Could you check a few things on this model? Use its own coordinates, in mm. Face numbers are marked on the shaded views. A direction names the side the tool comes from. Give positions to 0.01 mm unless a question says otherwise; leave off trailing zeros. Order: outer loops, then holes, each group sorted by start corner. A loop starts at its lowest first (then second) coordinate and runs counter-clockwise, first axis right, second up. Notation, with made-up numbers: (86, -8) -> (95, -8) arc R17 cw to (95, 13) -> close; hole circle Ø10 at (-38, 74.25). An arc over 180 degrees is marked (long way). Answer as CSV lines item,"result". Start each with the question number.
(1) I want a section at C-C (z = 21). Please give me the cut outline in (x, y), plus the area to 3 significant figures.
(2) We'd pull the mould along Z, two halves only. Please class the marked faces 3, 4, 5 and 6: released by +Z, released by -Z, zero draft, split by the parting line, or undercut.
(3) I want a section at A-A (y = 0). Please give me the cut outline in (x, z), plus the area to 3 significant figures.
(4) I need wall thicknesses on L1, parallel to Y at x = 0, z = 30.5; L2, parallel to Y at x = 0, z = 16; L3, parallel to Z at x = 14.5, y = -2.5. Which ranges of each line are inside material? Lowest first, please.
(5) I want a section at D-D (y = -11). Please give me the cut outline in (x, z), plus the area to 3 significant figures.
(6) Will these pins go through, and if not, where does the flat tip stop? pin 1 Ø5 at (y, z) = (8.5, 18.5) entering from +X; pin 2 Ø1.5 at (x, z) = (-8.5, 9.5) entering from +Y; pin 3 Ø1.5 at (x, z) = (6.5, 12.5) entering from +Y.
(7) On a 3-axis mill with a long thin cutter (end or side, diameter ignored), from which of +Z, -Z, +X, -X, +Y, -Y can I reach the whole of each face in a straight line? I mean the marked faces 1 and 2. Say none if no direction works.
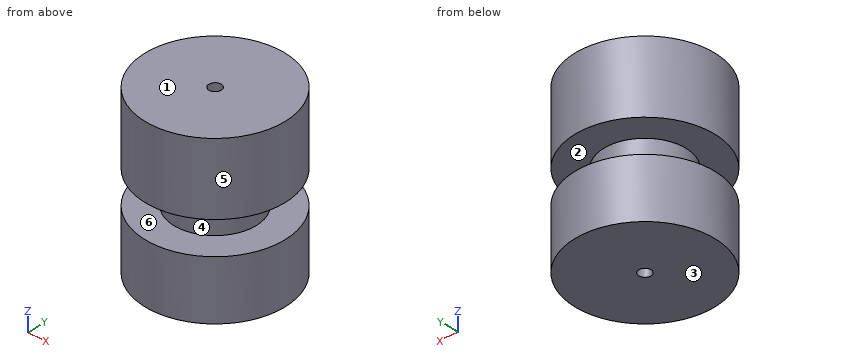
```python
from build123d import *

# Parameters (mm, degrees)
SKETCH1_R           = 17
SKETCH1_R_2         = 1.5
BOSS_EXTRUDE1_DEPTH = 40
CUT_EXTRUDE1_START  = -17.5
SKETCH2_R           = 17
SKETCH2_R_2         = 10
CUT_EXTRUDE1_DEPTH  = 8


with BuildPart() as part:
    # Sketch1 → Boss-Extrude1 (new body)
    with BuildSketch(Plane.XY):
        Circle(SKETCH1_R)
        Circle(SKETCH1_R_2, mode=Mode.SUBTRACT)
    extrude(amount=BOSS_EXTRUDE1_DEPTH)

    # Sketch2 → Cut-Extrude1 (cut)
    with BuildSketch(Plane.XY.offset(40).offset(CUT_EXTRUDE1_START)):
        Circle(SKETCH2_R)
        Circle(SKETCH2_R_2, mode=Mode.SUBTRACT)
    extrude(amount=-CUT_EXTRUDE1_DEPTH, mode=Mode.SUBTRACT)


solid = part.part
```
Final values:
1,outline,"circle Ø20 at (0, 0); hole circle Ø3 at (0, 0)"
1,area,"307 mm²"
2,face 3,"released by -Z"
2,face 4,"undercut"
2,face 5,"zero draft"
2,face 6,"undercut"
3,outline,"(-17, 0) -> (-1.5, 0) -> (-1.5, 40) -> (-17, 40) -> (-17, 22.5) -> (-10, 22.5) -> (-10, 14.5) -> (-17, 14.5) -> close; (1.5, 0) -> (17, 0) -> (17, 14.5) -> (10, 14.5) -> (10, 22.5) -> (17, 22.5) -> (17, 40) -> (1.5, 40) -> close"
3,area,"1,130 mm²"
4,L1,"-17 to -1.5, 1.5 to 17"
4,L2,"-10 to -1.5, 1.5 to 10"
4,L3,"0 to 14.5, 22.5 to 40"
5,outline,"(-12.96, 0) -> (12.96, 0) -> (12.96, 14.5) -> (-12.96, 14.5) -> close; (-12.96, 22.5) -> (12.96, 22.5) -> (12.96, 40) -> (-12.96, 40) -> close"
5,area,"830 mm²"
6,pin 1,"x = 8"
6,pin 2,"y = 15.13"
6,pin 3,"y = 16"
7,face 1,"+Z, +X, -X, +Y, -Y"
7,face 2,"none"
